```python
from build123d import *

# Parameters (mm, degrees)
SKETCH_1_W          = 230
SKETCH_1_H          = 150
EXTRUDE_1_DEPTH     = 3
SKETCH_7_R          = 2.6
CUT_EXTRUDE_4_DEPTH = 10
SKETCH1_R           = 1.6
CUT_EXTRUDE1_DEPTH  = 10


with BuildPart() as part:
    # 草图1 → 凸台-拉伸1 (new body)
    with BuildSketch(Plane.XY):
        with Locations((-30, 25)):
            Rectangle(SKETCH_1_W, SKETCH_1_H)
    extrude(amount=EXTRUDE_1_DEPTH)

    # 草图7 → 切除-拉伸4 (cut)
    with BuildSketch(Plane(origin=(0, 0, 0), x_dir=(-1, 0, 0), z_dir=(0, 0, -1))):
        with Locations((-20, 95)):
            Circle(SKETCH_7_R)
        with Locations((-72, 95)):
            Circle(SKETCH_7_R)
        with Locations((-46, 93)):
            Circle(SKETCH_7_R)
        with Locations((132, 95)):
            Circle(SKETCH_7_R)
        with Locations((106, 93)):
            Circle(SKETCH_7_R)
        with Locations((80, 95)):
            Circle(SKETCH_7_R)
    extrude(amount=-CUT_EXTRUDE_4_DEPTH, mode=Mode.SUBTRACT)

    # Sketch1 → Cut-Extrude1 (cut)
    with BuildSketch(Plane.XY.offset(3)):
        with Locations((-30, 36.5)):
            Circle(SKETCH1_R)
        with Locations((-11.5, 50)):
            Circle(SKETCH1_R)
        with Locations((-48.5, 50)):
            Circle(SKETCH1_R)
    extrude(amount=-CUT_EXTRUDE1_DEPTH, mode=Mode.SUBTRACT)


solid = part.part
```
Verification items for the finished model (mm, model axes). Coordinates: 2 decimals unless noted, no trailing zeros. Order: outer loops, then holes, each group sorted by start corner. A loop starts at its lowest first (then second) coordinate and runs counter-clockwise, first axis right, second up. Notation, with made-up numbers: (27, 31.5) - (35, 31.5) arc R14 ccw to (35, 39.5) - close; hole circle Ø3 at (-17, 51). An arc over 180 degrees is marked (long way). Return JSON: item names as keys, results as strings.
(1) Thickness scan on line 1 along Y through (x, z) = (-106, 1.45); line 2 along Y through (x, z) = (-11.5, 1.6). Record the ranges inside material, lowest first.
Filled sheet:
{"line 1": "y = -50 to 90.4, 95.6 to 100", "line 2": "y = -50 to 48.4, 51.6 to 100"}
(2) Mould release check, pull along Y, two halves, no side actions. Record for faces 1 (the flat face through (-32, 26, 3)), 2 (the cylindrical face through (-133.4, 97.19, 1.48)): pulls with the +Y half, pulls with the -Y half, needs draft (parallel to the pull), parting line crosses it, or undercut.
Filled sheet:
{"face 1": "needs draft", "face 2": "undercut"}
(3) Section check A-A, the plane x = 72. Record the cut outline in (y, z), and give its area (3 significant figures).
Filled sheet:
{"outline": "(-50, 0) - (92.4, 0) - (92.4, 3) - (-50, 3) - close; (97.6, 0) - (100, 0) - (100, 3) - (97.6, 3) - close", "area": "434 mm^2"}
(4) Go/stop test with a flat-tipped pin: pin 1 (4.5 mm diameter, centred on x = 46, y = 93, fed in from +Z). Record where the tip stops, or that it passes through.
Filled sheet:
{"pin 1": "passes through"}
